from build123d import *

# Parameters (mm, degrees)
F0_W     = 30
F0_H     = 30
F1_DEPTH = 30
F2_SIZE  = 10
F3_SIZE  = 10
F5_DEPTH = 27


with BuildPart() as f1:
    # F0 (on Top) → F1 (new body)
    with BuildSketch(Plane.XY):
        with Locations((15, 15)):
            Rectangle(F0_W, F0_H)
    extrude(amount=F1_DEPTH)

    # F2
    f2_edges = [f1.edges().sort_by_distance(p)[0] for p in [
        (0, 0, 15),
    ]]
    chamfer(f2_edges, length=F2_SIZE)

    # F3
    f3_edges = [f1.edges().sort_by_distance(p)[0] for p in [
        (20, 0, 30),
        (5, 5, 30),
        (0, 20, 30),
    ]]
    chamfer(f3_edges, length=F3_SIZE)

    # F4 (on face) → F5 (cut)
    with BuildSketch(Plane.XY.offset(30)):
        with BuildLine():
            Line((27, 27), (0, 27))
            ThreePointArc((0, 27), (-6.8211951152, -6.8211951152), (27, 0))
            Line((27, 0), (27, 27))
        make_face()
    extrude(amount=-F5_DEPTH, mode=Mode.SUBTRACT)


solid = f1.part
Could you check a few things on this model? Use its own coordinates, in mm. A direction names the side the tool comes from. Coordinates: 2 decimals unless noted, no trailing zeros. Loops run counter-clockwise (first coordinate to the right, second up) from the corner with the lowest first, then second, coordinate; pieces in that order, holes last. Notation, with made-up numbers: (19, -21) -> (42, -21) arc R16 cw to (42, 8) -> close; hole circle Ø10 at (51, -27.75). An arc over 180 degrees is marked (long way). Answer in a Markdown table with one row per item.
(1) Imagine slicing it at A-A (y = 7). List the corners of the cut face in (x, z) for me.
Results found:
| item | result |
|---|---|
| outline | (3, 0) -> (30, 0) -> (30, 27) -> (27, 27) -> (27, 3) -> (3, 3) -> close |
(2) For faces 1 (the face through (5, 28, 25)), 2 (the face through (13, 14, 3)), which set-ups out of +Z, -Z, +X, -X, +Y, -Y let a thin tool reach every point of the face, with its end or its side?
Results found:
| item | result |
|---|---|
| face 1 | +Z, -X, +Y, -Y |
| face 2 | +Z, -X, -Y |
(3) Imagine slicing it at B-B (z = 27.5). List the corners of the cut face in (x, y) for me.
Results found:
| item | result |
|---|---|
| outline | (7.5, 27) -> (27, 27) -> (27, 7.5) -> (30, 7.5) -> (30, 30) -> (7.5, 30) -> close |
(4) If I drill on probe 1 along Z at (x, y) = (11, 25.5); probe 2 along X at (y, z) = (17.75, 5), over which ranges is the centre line in solid material (lowest first)?
Results found:
| item | result |
|---|---|
| probe 1 | z = 0 to 3 |
| probe 2 | x = 27 to 30 |
(5) Will these pins go through, and if not, where does the flat tip stop? pin 1 Ø4 at (x, y) = (6.5, 4.5) entering from +Z; pin 2 Ø3 at (y, z) = (20, 18) entering from -X.
Results found:
| item | result |
|---|---|
| pin 1 | stops at z = 3 |
| pin 2 | stops at x = 27 |
